from build123d import *

# Parameters (mm, degrees)
F1_DEPTH = 50
F2_R     = 5
F3_DEPTH = 10
F4_R     = 5
F5_DEPTH = 10


with BuildPart() as f1:
    # F0 (on Front) → F1 (new body, symmetric)
    with BuildSketch(Plane.XZ):
        Polygon((0, 10), (0, 0), (50, 0), (50, 60), (40, 60), (40, 10), align=None)
    extrude(amount=F1_DEPTH, both=True)

    # F2 (on face) → F3 (cut, through all)
    with BuildSketch(Plane.YZ.offset(50)):
        with Locations((0, 40)):
            Circle(F2_R)
    extrude(amount=-F3_DEPTH, mode=Mode.SUBTRACT)

    # F4 (on face) → F5 (cut, through all)
    with BuildSketch(Plane.XY.offset(10)):
        with Locations((30, 0)):
            Circle(F4_R)
        with Locations((7.5, 13)):
            Circle(F4_R)
        with Locations((7.5, -13)):
            Circle(F4_R)
    extrude(amount=-F5_DEPTH, mode=Mode.SUBTRACT)


solid = f1.part
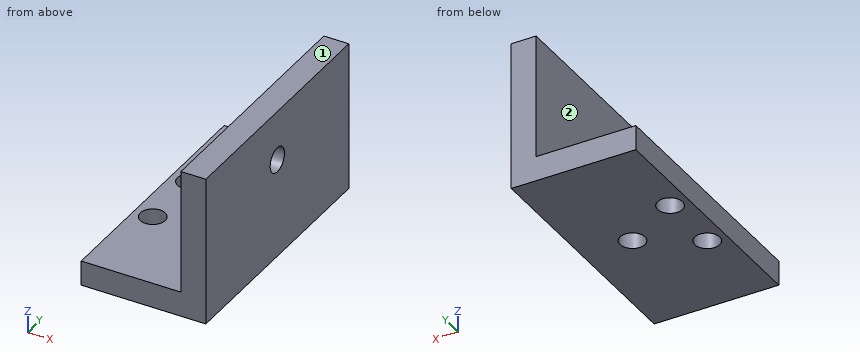
Check sheet for the modelled part. Datum: model origin and axes. Units: mm. Face numbers are marked on the shaded views. A direction names the side the tool comes from. Round coordinates to 2 decimals unless told otherwise and drop trailing zeros. Loops run counter-clockwise (first coordinate to the right, second up) from the corner with the lowest first, then second, coordinate; pieces in that order, holes last. Notation, with made-up numbers: (84, 34) -> (109, 34) arc R17 cw to (109, 49) -> close; hole circle Ø2 at (57, 22). An arc over 180 degrees is marked (long way). Put each result on its own line as item: value. Start each with the question number.
1. Section check C-C (x = 7.5). Enter the section's corners in (y, z), plus the area to 3 significant figures.
2. Section check B-B (y = 13). Enter the section's corners in (x, z).
3. Access from +Z, -Z, +X, -X, +Y, -Y to the whole of each face (thin tool, end or side, straight path). Record for the marked faces 1 and 2.
4. Section check A-A (z = 40). Enter the section's corners in (x, y), plus the area to 3 significant figures.
5. Gauge pin test, flat ends, axial feed: pin 1 (16 mm diameter, centred on x = 7.5, y = 13, fed in from +Z); pin 2 (10 mm diameter, centred on y = 19, z = 41, fed in from -X). Record the tip position at first contact, or that the pin passes through.
6. Scan lines: probe 1 along Y at (x, z) = (7.5, 2.75); probe 2 along Y at (x, z) = (30, 6); probe 3 along Z at (x, y) = (46.5, 0). Record each from-to range of solid material in increasing order.
7. Section check D-D (x = 30). Enter the section's corners in (y, z), plus the area to 3 significant figures.
Findings:
1. outline: (-50, 0) -> (-18, 0) -> (-18, 10) -> (-50, 10) -> close; (-8, 0) -> (8, 0) -> (8, 10) -> (-8, 10) -> close; (18, 0) -> (50, 0) -> (50, 10) -> (18, 10) -> close
1. area: 800 mm^2
2. outline: (0, 0) -> (2.5, 0) -> (2.5, 10) -> (0, 10) -> close; (12.5, 0) -> (50, 0) -> (50, 60) -> (40, 60) -> (40, 10) -> (12.5, 10) -> close
3. face 1: +Z, +X, -X, +Y, -Y
3. face 2: +Z, -X, +Y, -Y
4. outline: (40, -50) -> (50, -50) -> (50, -5) -> (40, -5) -> close; (40, 5) -> (50, 5) -> (50, 50) -> (40, 50) -> close
4. area: 900 mm^2
5. pin 1: stops at z = 10
5. pin 2: stops at x = 40
6. probe 1: y = -50 to -18, -8 to 8, 18 to 50
6. probe 2: y = -50 to -5, 5 to 50
6. probe 3: z = 0 to 35, 45 to 60
7. outline: (-50, 0) -> (-5, 0) -> (-5, 10) -> (-50, 10) -> close; (5, 0) -> (50, 0) -> (50, 10) -> (5, 10) -> close
7. area: 900 mm^2
